Can you work these out from the model? Positions are in its coordinate system, mm. A direction names the side the tool comes from. Coordinates: 2 decimals unless noted, no trailing zeros. Write each loop counter-clockwise with the first axis right and the second up, starting at its lowest first coordinate (ties: lowest second). Pieces come first, ordered by that corner, then holes. Notation, with made-up numbers: M 9,12 L 53,12 A16 ccw 53,28 Z; hole C 18,68 d1. An arc over 180 degrees is marked long. Use one line per item in the form item = value. Start each with the question number.
```python
from build123d import *

# Parameters (mm, degrees)
F0_W           = 50
F0_H           = 50
F1_DEPTH       = 50
F2_R           = 3
F3_T1_DEPTH    = 51.5
F3_T3_DEPTH    = 44
F3_T5_DEPTH    = 44
F3_S9_W        = 3.06
F3_S9_H        = 3.06
F3_T10_DEPTH   = 3.06
F3_S15_W       = 3.06
F3_S15_H       = 3.06
F3_T16_DEPTH   = 3.06
F3_S21_W       = 3.06
F3_S21_H       = 3.06
F3_T22_DEPTH   = 3.06
F3_S27_W       = 3.06
F3_S27_H       = 3.06
F3_T28_DEPTH   = 3.06
F5_DEPTH       = 10
F6_R           = 10
F7_DEPTH       = 10
F4_R           = 10
F8_DEPTH       = 20
F10_DEPTH      = 40
F10_DEPTH_BACK = 40
F11_R          = 10


# Not quite as in the source:
# - a fillet or chamfer that OpenCascade refuses, or shapes differently, is made with other operations: its cross-section is extruded or revolved along the edge and cut away or added


with BuildPart() as f1:
    # F0 (on Top) → F1 (new body)
    with BuildSketch(Plane.XY):
        Rectangle(F0_W, F0_H)
    extrude(amount=F1_DEPTH)

    # F2
    f2_edges = [f1.edges().sort_by_distance(p)[0] for p in [
        (25, 0, 50),
        (0, 25, 50),
        (-25, 0, 50),
        (0, -25, 50),
    ]]
    fillet(f2_edges, radius=F2_R)

    # F3: fillet of radius 3 on 12 edges, made by hand

    # F3_s2 → F3_t1 (cut)
    with BuildSketch(Plane.XY.offset(3)):
        with BuildLine():
            ThreePointArc((-22, -25), (-24.1213203436, -24.1213203436), (-25, -22))
            Line((-25, -22), (-25, -25))
            Line((-25, -25), (-22, -25))
        make_face()
        with BuildLine():
            ThreePointArc((25, -22), (24.1213203436, -24.1213203436), (22, -25))
            Line((22, -25), (25, -25))
            Line((25, -25), (25, -22))
        make_face()
        with BuildLine():
            ThreePointArc((25, 22), (24.1213203436, 24.1213203436), (22, 25))
            Line((22, 25), (25, 25))
            Line((25, 25), (25, 22))
        make_face()
        with BuildLine():
            ThreePointArc((-22, 25), (-24.1213203436, 24.1213203436), (-25, 22))
            Line((-25, 22), (-25, 25))
            Line((-25, 25), (-22, 25))
        make_face()
    extrude(amount=F3_T1_DEPTH, mode=Mode.SUBTRACT)

    # F3_s4 → F3_t3 (cut)
    with BuildSketch(Plane.YZ.offset(-22)):
        with BuildLine():
            ThreePointArc((-25, 3), (-24.1213203436, 0.8786796564), (-22, 0))
            Line((-22, 0), (-25, 0))
            Line((-25, 0), (-25, 3))
        make_face()
        with BuildLine():
            ThreePointArc((22, 0), (24.1213203436, 0.8786796564), (25, 3))
            Line((25, 3), (25, 0))
            Line((25, 0), (22, 0))
        make_face()
    extrude(amount=F3_T3_DEPTH, mode=Mode.SUBTRACT)

    # F3_s6 → F3_t5 (cut)
    with BuildSketch(Plane.XZ.offset(-22)):
        with BuildLine():
            ThreePointArc((25, 3), (24.1213203436, 0.8786796564), (22, 0))
            Line((22, 0), (25, 0))
            Line((25, 0), (25, 3))
        make_face()
        with BuildLine():
            ThreePointArc((-22, 0), (-24.1213203436, 0.8786796564), (-25, 3))
            Line((-25, 3), (-25, 0))
            Line((-25, 0), (-22, 0))
        make_face()
    extrude(amount=F3_T5_DEPTH, mode=Mode.SUBTRACT)


with BuildPart() as f3_tool8:
    # F3_s9 → F3_t10 (new body)
    with BuildSketch(Plane.XZ.offset(22)):
        with Locations((-23.53, 1.47)):
            Rectangle(F3_S9_W, F3_S9_H)
    extrude(amount=F3_T10_DEPTH)

    # F3_s11 → F3_t12 (revolve, cut)
    with BuildSketch(Plane(origin=(-22, -22, 3), x_dir=(0.7071067812, 0, 0.7071067812), z_dir=(0.7071067812, 0, -0.7071067812))):
        with BuildLine():
            ThreePointArc((0, -3), (3, 0), (0, 3))
            Line((0, 3), (0, -3))
        make_face()
    revolve(axis=Axis((-22, -22, 3), (0, -1, 0)), mode=Mode.SUBTRACT)


with BuildPart() as f1_1:
    add(f1.part)

    # F3_t7: cut F3_tool8
    add(f3_tool8.part, mode=Mode.SUBTRACT)


with BuildPart() as f3_tool14:
    # F3_s15 → F3_t16 (new body)
    with BuildSketch(Plane.YZ.offset(22)):
        with Locations((-23.53, 1.47)):
            Rectangle(F3_S15_W, F3_S15_H)
    extrude(amount=F3_T16_DEPTH)

    # F3_s17 → F3_t18 (revolve, cut)
    with BuildSketch(Plane(origin=(22, -22, 3), x_dir=(0, 0.7071067812, 0.7071067812), z_dir=(0, 0.7071067812, -0.7071067812))):
        with BuildLine():
            ThreePointArc((0, -3), (3, 0), (0, 3))
            Line((0, 3), (0, -3))
        make_face()
    revolve(axis=Axis((22, -22, 3), (1, 0, 0)), mode=Mode.SUBTRACT)


with BuildPart() as f1_2:
    add(f1_1.part)

    # F3_t13: cut F3_tool14
    add(f3_tool14.part, mode=Mode.SUBTRACT)


with BuildPart() as f3_tool20:
    # F3_s21 → F3_t22 (new body)
    with BuildSketch(Plane.YZ.offset(22)):
        with Locations((23.53, 1.47)):
            Rectangle(F3_S21_W, F3_S21_H)
    extrude(amount=F3_T22_DEPTH)

    # F3_s23 → F3_t24 (revolve, cut)
    with BuildSketch(Plane(origin=(22, 22, 3), x_dir=(0, -0.7071067812, 0.7071067812), z_dir=(0, 0.7071067812, 0.7071067812))):
        with BuildLine():
            ThreePointArc((0, -3), (3, 0), (0, 3))
            Line((0, 3), (0, -3))
        make_face()
    revolve(axis=Axis((22, 22, 3), (1, 0, 0)), mode=Mode.SUBTRACT)


with BuildPart() as f1_3:
    add(f1_2.part)

    # F3_t19: cut F3_tool20
    add(f3_tool20.part, mode=Mode.SUBTRACT)


with BuildPart() as f3_tool26:
    # F3_s27 → F3_t28 (new body)
    with BuildSketch(Plane.XY.offset(3)):
        with Locations((-23.53, 23.53)):
            Rectangle(F3_S27_W, F3_S27_H)
    extrude(amount=-F3_T28_DEPTH)

    # F3_s29 → F3_t30 (revolve, cut)
    with BuildSketch(Plane(origin=(-22, 22, 3), x_dir=(0.7071067812, -0.7071067812, 0), z_dir=(0.7071067812, 0.7071067812, 0))):
        with BuildLine():
            ThreePointArc((0, -3), (3, 0), (0, 3))
            Line((0, 3), (0, -3))
        make_face()
    revolve(axis=Axis((-22, 22, 3), (0, 0, -1)), mode=Mode.SUBTRACT)


with BuildPart() as f1_4:
    add(f1_3.part)

    # F3_t25: cut F3_tool26
    add(f3_tool26.part, mode=Mode.SUBTRACT)

    # F5 (cut): a face of the model
    f5_faces = [f1_4.faces().sort_by_distance(p)[0] for p in [
        (0, 0, 0),
    ]]
    extrude(f5_faces, amount=-F5_DEPTH, mode=Mode.SUBTRACT)

    # F6 (on face) → F7 (cut)
    with BuildSketch(Plane.YZ.offset(25)):
        with Locations((0, 25)):
            Circle(F6_R)
    extrude(amount=-F7_DEPTH, mode=Mode.SUBTRACT)

    # F4 (on face) → F8 (join)
    with BuildSketch(Plane(origin=(-25, 0, 0), x_dir=(0, -1, 0), z_dir=(-1, 0, 0))):
        with Locations((0, 25)):
            Circle(F4_R)
    extrude(amount=F8_DEPTH)

    # F9 (on Front) → F10 (join, two sides)
    with BuildSketch(Plane.XZ) as f10_sk:
        Polygon((21, 55.5713325143), (21, 66.5713325143), (-52, 66.5713325143), (-52, -196.4604258537), (-32, -196.4604258537), (-32, 55.5713325143), align=None)
    extrude(amount=F10_DEPTH)
    extrude(f10_sk.sketch, amount=-F10_DEPTH_BACK)

    # F11
    f11_edges = [f1_4.edges().sort_by_distance(p)[0] for p in [
        (-52, 0, 66.571333),
    ]]
    fillet(f11_edges, radius=F11_R)


solid = f1_4.part
```
1) Suppose I cut it at A-A on y = 17. Please give me the cut outline in (x, z), and give its area (3 significant figures).
2) Will these pins go through, and if not, where does the flat tip stop? pin 1 Ø22 at (x, z) = (-10.5, 33.5) entering from -Y; pin 2 Ø12 at (x, z) = (-30, -93) entering from +Y; pin 3 Ø16 at (x, y) = (-7, -18.5) entering from -Z; pin 4 Ø1.5 at (y, z) = (-32, -45) entering from +X.
3) Which directions (+Z, -Z, +X, -X, +Y, -Y) give clear straight access to the entire face, cutting with the end or side of a thin tool? Please do faces 5 (the face through (0, 0, 50)), 6 (the face through (-22, 0, 5)), 7 (the face through (0, -25, 25)), 8 (the face through (0, 25, 25)).
4) Suppose I cut it at D-D on y = 0. Please give me the cut outline in (x, z), and give its area (3 significant figures).
5) Suppose I cut it at C-C on z = 25. Please give me the cut outline in (x, y).
6) Please list where these lines run through material, in increasing order: line 1 (Z direction, x = 18, y = 0.5); line 2 (X direction, y = 18.5, z = 9.5); line 3 (Z direction, x = 21.5, y = 0).
7) If we mould it in two halves opening along Z, with no side actions, what happens to faces 1 (the face through (-10, -1, 66.571)), 2 (the face through (-28.451, 1.302, 34.915)), 3 (the face through (-37, -40, -55)), 4 (the face through (0, 0, 10))? For each: +Z half, -Z half, draft (parallel to the pull), parting line (faces both ways), or undercut.
8) Suppose I cut it at B-B on x = -5.5. Please give me the cut outline in (y, z).
Computed values:
q1.outline = M -52,-196.46 L -32,-196.46 L -32,55.57 L 21,55.57 L 21,66.57 L -42,66.57 A10 ccw -52,56.57 Z; M -25,3 A3 ccw -22,0 L -22,10 L 22,10 L 22,0 A3 ccw 25,3 L 25,47 A3 ccw 22,50 L -22,50 A3 ccw -25,47 Z
q1.area = 7,870 mm²
q2.pin_1 = -25
q2.pin_2 = 40
q2.pin_3 = 0
q2.pin_4 = -32
q3.face_5 = +X, +Y, -Y
q3.face_6 = -Z
q3.face_7 = -Z, +X, -Y
q3.face_8 = -Z, +X, +Y
q4.outline = M -52,-196.46 L -32,-196.46 L -32,15 L -25,15 L -25,3 A3 ccw -22,0 L -22,10 L 22,10 L 22,0 A3 ccw 25,3 L 25,15 L 15,15 L 15,35 L 25,35 L 25,47 A3 ccw 22,50 L -22,50 A3 ccw -25,47 L -25,35 L -32,35 L -32,55.57 L 21,55.57 L 21,66.57 L -42,66.57 A10 ccw -52,56.57 Z
q4.area = 7,810 mm²
q5.outline = M -52,-40 L -32,-40 L -32,-10 L -25,-10 L -25,-22 A3 ccw -22,-25 L 22,-25 A3 ccw 25,-22 L 25,-10 L 15,-10 L 15,10 L 25,10 L 25,22 A3 ccw 22,25 L -22,25 A3 ccw -25,22 L -25,10 L -32,10 L -32,40 L -52,40 Z
q6.line_1 = 10 to 15.01, 34.99 to 50, 55.57 to 66.57
q6.line_2 = -52 to -32, -25 to -22, 22 to 25
q6.line_3 = 10 to 15, 35 to 50
q7.face_1 = +Z half
q7.face_2 = undercut
q7.face_3 = draft
q7.face_4 = -Z half
q8.outline = M -40,55.57 L 40,55.57 L 40,66.57 L -40,66.57 Z; M -25,3 A3 ccw -22,0 L -22,10 L 22,10 L 22,0 A3 ccw 25,3 L 25,47 A3 ccw 22,50 L -22,50 A3 ccw -25,47 Z
